Read the model definition and answer for the solid it produces. Units are mm, in the model's axes. A direction names the side the tool comes from. Give positions to 0.01 mm unless a question says otherwise; leave off trailing zeros. Order: outer loops, then holes, each group sorted by start corner. A loop starts at its lowest first (then second) coordinate and runs counter-clockwise, first axis right, second up. Notation, with made-up numbers: (13.5, -20) - (27.5, -20) arc R14 cw to (27.5, 1) - close; hole circle Ø10 at (59, 49.25). An arc over 180 degrees is marked (long way). Answer as CSV lines item,"result". Start each with the question number.
from build123d import *

# Parameters (mm, degrees)
SKETCH1_W           = 90
SKETCH1_H           = 95
BOSS_EXTRUDE1_DEPTH = 3
SKETCH4_W           = 3
SKETCH4_H           = 15
BOSS_EXTRUDE4_DEPTH = 3
SKETCH5_W           = 90
SKETCH5_H           = 3
BOSS_EXTRUDE5_DEPTH = 3
SKETCH6_W           = 40
SKETCH6_H           = 3
CUT_EXTRUDE2_DEPTH  = 4
SKETCH8_R           = 8.15
CUT_EXTRUDE3_DEPTH  = 4


with BuildPart() as part:
    # Sketch1 → Boss-Extrude1 (new body)
    with BuildSketch(Plane(origin=(0, 0, 0), x_dir=(1, 0, 0), z_dir=(0, 1, 0))):
        with Locations((45, 47.5)):
            Rectangle(SKETCH1_W, SKETCH1_H)
    extrude(amount=BOSS_EXTRUDE1_DEPTH)

    # Sketch4 → Boss-Extrude4 (add)
    with BuildSketch(Plane(origin=(0, 3, 0), x_dir=(1, 0, 0), z_dir=(0, 1, 0))):
        with Locations((-1.5, 77.5)):
            Rectangle(SKETCH4_W, SKETCH4_H)
        with Locations((-1.5, 47.5)):
            Rectangle(SKETCH4_W, SKETCH4_H)
        with Locations((-1.5, 17.5)):
            Rectangle(SKETCH4_W, SKETCH4_H)
        with Locations((91.5, 77.5)):
            Rectangle(SKETCH4_W, SKETCH4_H)
        with Locations((91.5, 47.5)):
            Rectangle(SKETCH4_W, SKETCH4_H)
        with Locations((91.5, 17.5)):
            Rectangle(SKETCH4_W, SKETCH4_H)
    extrude(amount=-BOSS_EXTRUDE4_DEPTH)

    # Sketch5 → Boss-Extrude5 (add)
    with BuildSketch(Plane(origin=(0, 3, 0), x_dir=(1, 0, 0), z_dir=(0, 1, 0))):
        with Locations((45, 96.5)):
            Rectangle(SKETCH5_W, SKETCH5_H)
    extrude(amount=-BOSS_EXTRUDE5_DEPTH)

    # Sketch6 → Cut-Extrude2 (cut)
    with BuildSketch(Plane(origin=(0, 3, 0), x_dir=(1, 0, 0), z_dir=(0, 1, 0))):
        with Locations((45, 96.5)):
            Rectangle(SKETCH6_W, SKETCH6_H)
    extrude(amount=-CUT_EXTRUDE2_DEPTH, mode=Mode.SUBTRACT)

    # Sketch8 → Cut-Extrude3 (cut, through all)
    with BuildSketch(Plane(origin=(0, 3, 0), x_dir=(1, 0, 0), z_dir=(0, 1, 0))):
        with Locations((32.31, 47.5)):
            Circle(SKETCH8_R)
        with Locations((57.69, 47.5)):
            Circle(SKETCH8_R)
    extrude(amount=-CUT_EXTRUDE3_DEPTH, mode=Mode.SUBTRACT)


solid = part.part
(1) Section B-B, the plane z = -47.5 is taken. Write down the section's boundary in (x, y).
(2) Section D-D, the plane z = -67 is taken. Write down the section's boundary in (x, y), and give its area (3 significant figures).
(3) Flat-ended cylindrical pins translate along their axes: pin 1 Ø0.9 at (y, z) = (2, -90.5) entering from +X; pin 2 Ø14.5 at (x, z) = (57.69, -47.5) entering from +Y; pin 3 Ø0.9 at (y, z) = (1, -7) entering from -X. Find the tip coordinate at first contact, or state that the pin passes through.
(4) Section A-A, the plane x = 32.31 is taken. Write down the section's boundary in (y, z), and give its area (3 significant figures).
(5) Determine the mould class of faces 5 (the flat face through (0, 1, -62)), 6 (the flat face through (-3, 2, -77)), 7 (the flat face through (12, 2, -98)) for opening direction Z: released by +Z, released by -Z, zero draft, split by the parting line, or undercut.
(6) Which of the six approach directions +Z, -Z, +X, -X, +Y, -Y give full straight-line access (tool end or side, diameter ignored) to faces 1 (the flat face through (93, 2, -17)), 2 (the flat face through (90, 1, -62)), 3 (the flat face through (25, 2, -96)), 4 (the flat face through (-2, 2, -40))?
(7) Straight lines are drawn through the part: line 1 (X direction, y = 2.45, z = -47.5); line 2 (X direction, y = 1.7, z = -50); line 3 (Z direction, x = 57.69, y = 0.95). For each, find the intervals that lie inside material, in ascending order. Write a range as [from, to].
(8) Section C-C, the plane y = 0.9 is taken. State how many separate pieces and enclosed holes the cut face has, and give its area (3 significant figures).
Checks:
1,outline,"(-3, 0) - (24.16, 0) - (24.16, 3) - (-3, 3) - close; (40.46, 0) - (49.54, 0) - (49.54, 3) - (40.46, 3) - close; (65.84, 0) - (93, 0) - (93, 3) - (65.84, 3) - close"
2,outline,"(0, 0) - (90, 0) - (90, 3) - (0, 3) - close"
2,area,"270 mm²"
3,pin 1,"stops at x = 90"
3,pin 2,"passes through"
3,pin 3,"stops at x = 0"
4,outline,"(0, -95) - (3, -95) - (3, -55.65) - (0, -55.65) - close; (0, -39.35) - (3, -39.35) - (3, 0) - (0, 0) - close"
4,area,"236 mm²"
5,face 5,"undercut"
5,face 6,"zero draft"
5,face 7,"released by -Z"
6,face 1,"+Z, -Z, +X, +Y, -Y"
6,face 2,"+X, +Y, -Y"
6,face 3,"-Z, +Y, -Y"
6,face 4,"-X, +Y, -Y"
7,line 1,"x = [-3, 24.16], [40.46, 49.54], [65.84, 93]"
7,line 2,"x = [-3, 24.55], [40.07, 49.93], [65.45, 93]"
7,line 3,"z = [-95, -55.65], [-39.35, 0]"
8,separate pieces,"1"
8,enclosed holes,"2"
8,area,"8,550 mm²"
